Build history of the part. All positions in model axes, mm. A direction names the side the tool comes from. Round coordinates to 2 decimals unless told otherwise and drop trailing zeros. Order: outer loops, then holes, each group sorted by start corner. A loop starts at its lowest first (then second) coordinate and runs counter-clockwise, first axis right, second up. Notation, with made-up numbers: M 40.25,-2 L 86.25,-2 A20 cw 86.25,25 Z; hole C 44.5,75 d10. An arc over 180 degrees is marked long. One line per item, written item: value. Start each with the question number.
Item 1: Band-saw the part on A-A, the plane x = -21. Write the cut outline in (y, z) (3 decimals), then the cut area to 3 significant figures.
Item 2: Band-saw the part on B-B, the plane y = -21.5. Write the cut outline in (x, z) (3 decimals), then the cut area to 3 significant figures.
Item 3: Probe L1, parallel to X at y = -14, z = -5 (3 decimals); L2, parallel to Y at x = -34, z = 6; L3, parallel to Z at x = 21, y = 0.5 (3 decimals). List the from-to ranges inside material, lowest first.
Item 4: Band-saw the part on C-C, the plane y = 16. Write the cut outline in (x, z) (3 decimals), then the cut area to 3 significant figures.
Item 5: Tool access for faces 1 (the flat face through (0, 0, -8)), 2 (the flat face through (0, 13, -6.35)), 3 (the flat face through (0, 7, 9.525)): list every direction of +Z, -Z, +X, -X, +Y, -Y with a clear straight run to the whole face (end or side of a thin tool).
Item 6: Two-plate mould, pull along X, no slides. Class faces 4 (the flat face through (34.925, -28, 3)), 5 (the flat face through (0, 13, 6.35)), 6 (the cylindrical face through (-33.32, -64.53, 4.01)): +X half, -X half, draft (parallel to the pull), parting line (faces both ways), or undercut.
Item 7: Pin check, flat tips, straight feed: pin 1 (5 mm diameter, centred on y = -24.5, z = 13, fed in from -X); pin 2 (7.5 mm diameter, centred on x = 12.5, y = 9.5, fed in from +Z) (3 decimals); pin 3 (3.5 mm diameter, centred on x = -16, z = -7, fed in from -Y). Stop position of each tip, or through.
```python
from build123d import *

# Parameters (mm, degrees)
PROBEPROFILE_W      = 69.85
PROBEPROFILE_H      = 19.05
PROBEPROFILE_W_2    = 63.5
PROBEPROFILE_H_2    = 12.7
EXTRUDE_THIN1_DEPTH = 25.4
SKETCH2_R           = 15.875
BOSS_EXTRUDE1_DEPTH = 34.925
SKETCH2_2_R         = 15.875
CUT_EXTRUDE1_DEPTH  = 31.75
SKETCH3_W           = 3.175
SKETCH3_H           = 19.05
BOSS_EXTRUDE2_DEPTH = 66.675
CUT_EXTRUDE2_START  = -69.85
SKETCH4_R           = 3.175
CUT_EXTRUDE2_DEPTH  = 69.85


with BuildPart() as part:
    # ProbeProfile → Extrude-Thin1 (new body)
    with BuildSketch(Plane(origin=(0, 0, 0), x_dir=(1, 0, 0), z_dir=(0, 1, 0))):
        Rectangle(PROBEPROFILE_W, PROBEPROFILE_H)
        Rectangle(PROBEPROFILE_W_2, PROBEPROFILE_H_2, mode=Mode.SUBTRACT)
    extrude(amount=EXTRUDE_THIN1_DEPTH)



with BuildPart() as body_2:
    # Sketch2 → Boss-Extrude1 (new body, symmetric)
    with BuildSketch(Plane(origin=(0, 0, 0), x_dir=(0, 0, -1), z_dir=(1, 0, 0))):
        with Locations((-6.35, -66.675)):
            Circle(SKETCH2_R)
    extrude(amount=BOSS_EXTRUDE1_DEPTH, both=True)

    # Sketch2<2> → Cut-Extrude1 (cut, symmetric)
    with BuildSketch(Plane(origin=(0, 0, 0), x_dir=(0, 0, -1), z_dir=(1, 0, 0))):
        with Locations((-6.35, -66.675)):
            Circle(SKETCH2_2_R)
    extrude(amount=CUT_EXTRUDE1_DEPTH, both=True, mode=Mode.SUBTRACT)


with BuildPart() as part_1:
    add(part.part)

    add(body_2.part)  # Boss-Extrude2 merges body 2
    # Sketch3 → Boss-Extrude2 (add)
    with BuildSketch(Plane.XZ):
        with Locations((33.3375, 0)):
            Rectangle(SKETCH3_W, SKETCH3_H)
        with Locations((-33.3375, 0)):
            Rectangle(SKETCH3_W, SKETCH3_H)
    extrude(amount=BOSS_EXTRUDE2_DEPTH)

    # Sketch4 → Cut-Extrude2 (cut)
    with BuildSketch(Plane.ZY.offset(34.925).offset(CUT_EXTRUDE2_START)):
        with Locations((6.35, -66.675)):
            Circle(SKETCH4_R)
    extrude(amount=CUT_EXTRUDE2_DEPTH, mode=Mode.SUBTRACT)


solid = part_1.part
```
Output:
1. outline: M 0,-9.525 L 25.4,-9.525 L 25.4,-6.35 L 0,-6.35 Z; M 0,6.35 L 25.4,6.35 L 25.4,9.525 L 0,9.525 Z
1. area: 161 mm²
2. outline: M -34.925,-9.525 L -31.75,-9.525 L -31.75,9.525 L -34.925,9.525 Z; M 31.75,-9.525 L 34.925,-9.525 L 34.925,9.525 L 31.75,9.525 Z
2. area: 121 mm²
3. L1: x = -34.925 to -31.75, 31.75 to 34.925
3. L2: y = -82.55 to -69.83, -63.52 to 25.4
3. L3: z = -9.525 to -6.35, 6.35 to 9.525
4. outline: M -34.925,-9.525 L 34.925,-9.525 L 34.925,9.525 L -34.925,9.525 Z; hole M -31.75,-6.35 L 31.75,-6.35 L 31.75,6.35 L -31.75,6.35 Z
4. area: 524 mm²
5. face 1: +Z, -Z, -Y
5. face 2: +Y, -Y
5. face 3: +Z, +X, -X, +Y
6. face 4: +X half
6. face 5: undercut
6. face 6: draft
7. pin 1: passes through
7. pin 2: stops at z = 9.525
7. pin 3: stops at y = 0
